Study the drawing (mm; zero at the part's minimum x, y, z) and answer. Round coordinates to 2 decimals unless told otherwise and drop trailing zeros. Loops run counter-clockwise (first coordinate to the right, second up) from the corner with the lowest first, then second, coordinate; pieces in that order, holes last. Notation, with made-up numbers: M -28.75,28.25 L 12.25,28.25 A12 ccw 12.25,34.25 Z; hole C 15.25,79.5 d1. An arc over 180 degrees is marked long. Write each question's results on one line, items separated by ' | '.
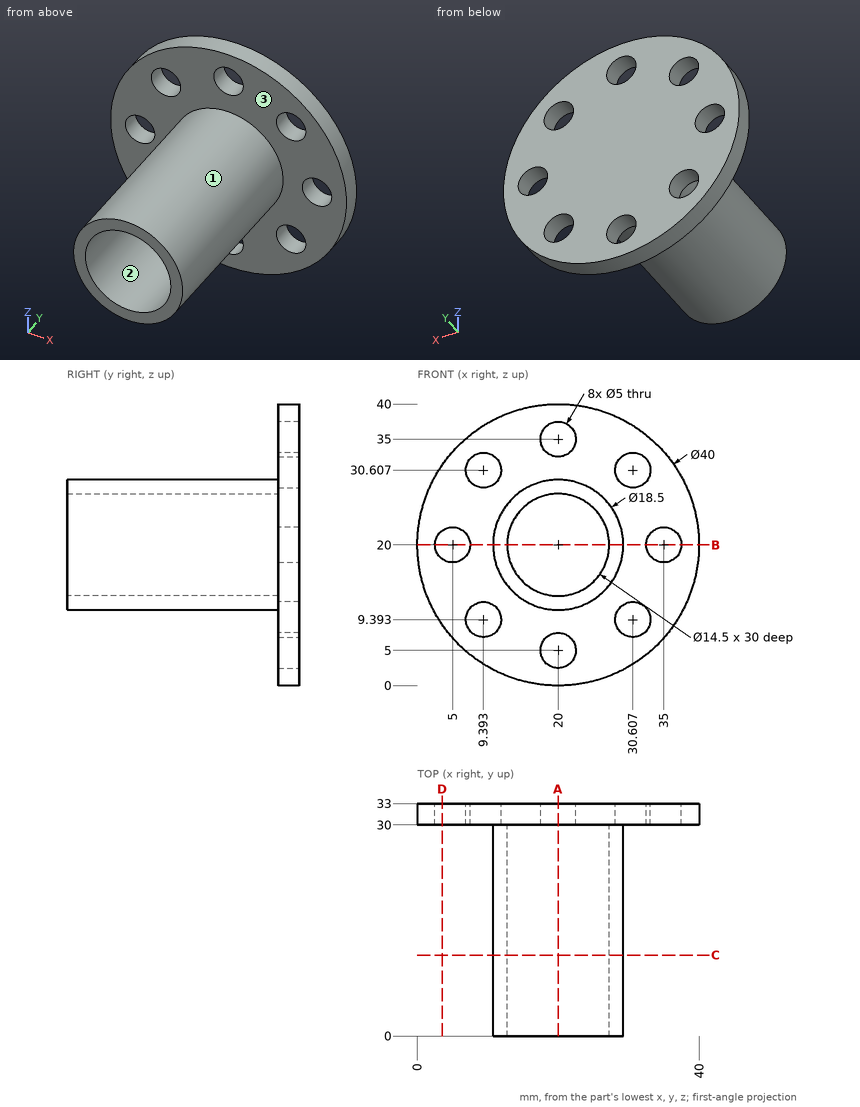
Item 1: Straight lines are drawn through the part: line 1 (X direction, y = 30.75, z = 20); line 2 (Z direction, x = 19.5, y = 31.5); line 3 (Z direction, x = 23.5, y = 1). For each, find the intervals that lie inside material, in ascending order.
Outcome:
line 1: x = 0 to 2.5, 7.5 to 32.5, 37.5 to 40 | line 2: z = 0.01 to 2.55, 7.45 to 32.55, 37.45 to 39.99 | line 3: z = 11.44 to 13.65, 26.35 to 28.56
Item 2: The part is cut by section A-A (x = 20). Determine the outline of the cut face in (y, z).
Outcome:
outline: M 0,10.75 L 30,10.75 L 30,7.5 L 33,7.5 L 33,32.5 L 30,32.5 L 30,29.25 L 0,29.25 L 0,27.25 L 30,27.25 L 30,12.75 L 0,12.75 Z; M 30,0 L 33,0 L 33,2.5 L 30,2.5 Z; M 30,37.5 L 33,37.5 L 33,40 L 30,40 Z
Item 3: Flat-ended cylindrical pins translate along their axes: pin 1 (4 mm diameter, centred on x = 20, z = 35, fed in from +Y); pin 2 (12 mm diameter, centred on y = 28, z = 18, fed in from -X); pin 3 (10 mm diameter, centred on x = 13, y = 11, fed in from +Z); pin 4 (12 mm diameter, centred on y = 11, z = 5.5, fed in from -X). Find the tip coordinate at first contact, or state that the pin passes through.
Outcome:
pin 1: passes through | pin 2: stops at x = 0 | pin 3: stops at z = 29.03 | pin 4: stops at x = 16.35
Item 4: The part is cut by section D-D (x = 3.5). Determine the outline of the cut face in (y, z).
Outcome:
outline: M 30,8.7 L 33,8.7 L 33,18 L 30,18 Z; M 30,22 L 33,22 L 33,31.3 L 30,31.3 Z
Item 5: The part is cut by section B-B (z = 20). Determine the outline of the cut face in (x, y).
Outcome:
outline: M 0,30 L 2.5,30 L 2.5,33 L 0,33 Z; M 7.5,30 L 10.75,30 L 10.75,0 L 12.75,0 L 12.75,30 L 27.25,30 L 27.25,0 L 29.25,0 L 29.25,30 L 32.5,30 L 32.5,33 L 7.5,33 Z; M 37.5,30 L 40,30 L 40,33 L 37.5,33 Z
Item 6: The part is cut by section C-C (y = 11.5). Determine the outline of the cut face in (x, z), plus the area to 3 significant figures.
Outcome:
outline: C 20,20 d18.5; hole C 20,20 d14.5 | area: 104 mm2
Item 7: The mould has two halves that part along X. Classify the marked faces 1, 2 and 3: pulls with the +X half, pulls with the -X half, needs draft (parallel to the pull), parting line crosses it, or undercut.
Outcome:
face 1: parting line crosses it | face 2: undercut | face 3: needs draft
